Can you work these out from the model? Positions are in its coordinate system, mm. Face numbers are marked on the shaded views. A direction names the side the tool comes from. Give positions to 0.01 mm unless a question says otherwise; leave off trailing zeros. Order: outer loops, then holes, each group sorted by start corner. A loop starts at its lowest first (then second) coordinate and runs counter-clockwise, first axis right, second up. Notation, with made-up numbers: (68, -25) - (89, -25) arc R18 ccw to (89, -14) - close; hole circle Ø5 at (-21.75, 55). An arc over 180 degrees is marked (long way). Return JSON: item names as keys, results as strings.
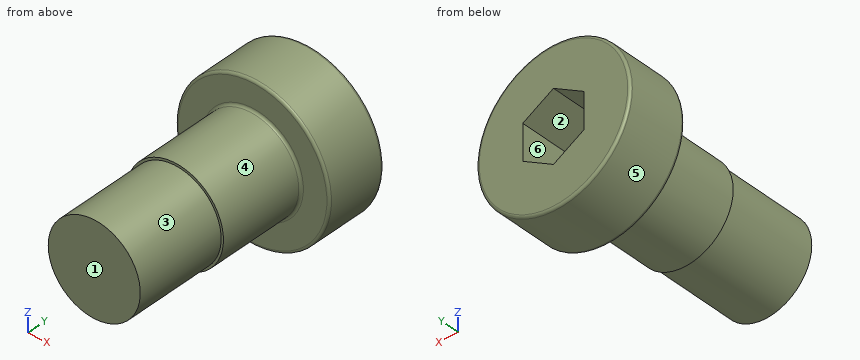
```python
from build123d import *

# Parameters (mm, degrees)
SKETCH1_W          = 4.7625
SKETCH1_H          = 9.525
CUT_EXTRUDE1_DEPTH = 6.35
FILLET1_R          = 0.254
FILLET2_R          = 0.254


with BuildPart() as part:
    # Sketch1 → Revolve1 (revolve)
    with BuildSketch(Plane.XY, mode=Mode.PRIVATE) as revolve1_sk:
        with Locations((2.38125, -9.32561)):
            Rectangle(SKETCH1_W, SKETCH1_H)
        Polygon((4.7625, -4.56311), (5, -4.56311), (5, 4.56311), (0, 4.56311), (0, -4.56311), align=None)
        Polygon((0, 4.56311), (5, 4.56311), (7.9375, 4.56311), (7.9375, 10.91311), (0, 10.91311), align=None)
    revolve(revolve1_sk.sketch.rotate(Axis((0, -16.678845395, 0), (0, -1, 0)), 180), axis=Axis((0, -16.678845395, 0), (0, -1, 0)))

    # Sketch2 → Cut-Extrude1 (cut)
    with BuildSketch(Plane(origin=(0, 10.91311, 0), x_dir=(1, 0, 0), z_dir=(0, 1, 0))):
        Polygon((0, 3.666174209), (-3.175, 1.833087105), (-3.175, -1.833087105), (0, -3.666174209), (3.175, -1.833087105), (3.175, 1.833087105), align=None)
    extrude(amount=-CUT_EXTRUDE1_DEPTH, mode=Mode.SUBTRACT)

    # Fillet1
    fillet1_edges = [part.edges().sort_by_distance(p)[0] for p in [
        (5, 4.56311, 0),
    ]]
    fillet(fillet1_edges, radius=FILLET1_R)

    # Fillet2
    fillet2_edges = [part.edges().sort_by_distance(p)[0] for p in [
        (7.9375, 10.91311, 0),
        (7.9375, 4.56311, 0),
    ]]
    fillet(fillet2_edges, radius=FILLET2_R)


solid = part.part
```
1. On a 3-axis mill with a long thin cutter (end or side, diameter ignored), from which of +Z, -Z, +X, -X, +Y, -Y can I reach the whole of each face in a straight line? I mean the marked faces 4, 5 and 6. Say none if no direction works.
Checks:
{"face 4": "-Y", "face 5": "+Y, -Y", "face 6": "+Y"}
2. Suppose I cut it at C-C (y = -10.5). List the corners of the cut face in (x, z) for me (1 decimal), plus the area to 3 significant figures.
Checks:
{"outline": "circle Ø9.5 at (0, 0)", "area": "71.3 mm^2"}
3. For pin 1 Ø3 at (y, z) = (3, 5) entering from -X; pin 2 Ø4 at (y, z) = (-5.5, -3) entering from +X; pin 3 Ø6 at (x, y) = (6, -6.5) entering from -Z, each with a flat end and sliding along its axis, tell me the tip position at first contact or that it passes through.
Checks:
{"pin 1": "x = -3.57", "pin 2": "x = 4.85", "pin 3": "z = -3.7"}
4. If I drill on L1, parallel to Y at x = -1.75, z = -6; L2, parallel to Z at x = -0.25, y = -7.25; L3, parallel to Z at x = 2.5, y = 5.5, over which ranges is the centre line in solid material (lowest first)? Write a range as [from, to].
Checks:
{"L1": "[4.56, 10.91]", "L2": "[-4.76, 4.76]", "L3": "[-7.53, -2.22], [2.22, 7.53]"}
5. Suppose I cut it at B-B (y = -2.5). List the corners of the cut face in (x, z) for me.
Checks:
{"outline": "circle Ø10 at (0, 0)"}
6. Thinking about a two-plate mould opening in Z: for the marked faces 1, 2 and 3, which applies, +Z half, -Z half, draft (parallel to the pull), parting line (faces both ways), or undercut?
Checks:
{"face 1": "draft", "face 2": "undercut", "face 3": "parting line"}
